```python
from build123d import *

# Parameters (mm, degrees)
SKETCH_3_W           = 10
SKETCH_3_H           = 40
SKETCH_3_W_2         = 25.75
SKETCH_3_H_2         = 10
SKETCH_3_W_3         = 36.25
SKETCH_3_W_4         = 25
EXTRUDE_1_DEPTH      = 1
EXTRUDE_2_DEPTH      = 4
EXTRUDE_2_DEPTH_BACK = 1
SKETCH_5_W           = 25
SKETCH_5_H           = 10
SKETCH_5_W_2         = 10
SKETCH_5_H_2         = 40
EXTRUDE_3_DEPTH      = 2


with BuildPart() as part:
    # 草图3 → 凸台-拉伸1 (new body)
    with BuildSketch(Plane(origin=(0, 0, 0), x_dir=(1, 0, 0), z_dir=(0, 1, 0))):
        with Locations((20, 0)):
            Rectangle(SKETCH_3_W, SKETCH_3_H)
        with Locations((2.125, 0)):
            Rectangle(SKETCH_3_W_2, SKETCH_3_H_2)
        Polygon((-10.75, -5), (-10.75, 5), (-10.75, 25), (-20.75, 25), (-20.75, 5), (-20.75, -5), (-20.75, -25), (-10.75, -25), align=None)
        with Locations((-38.875, 0)):
            Rectangle(SKETCH_3_W_3, SKETCH_3_H_2)
        with Locations((-69.5, 0)):
            Rectangle(SKETCH_3_W_4, SKETCH_3_H_2)
    extrude(amount=EXTRUDE_1_DEPTH)

    # 草图4 → 凸台-拉伸2 (add, two sides)
    with BuildSketch(Plane.XZ) as extrude_2_sk:
        Polygon((14, -21), (26, -21), (26, 21), (14, 21), (14, 6), (-9.75, 6), (-9.75, 26), (-21.75, 26), (-21.75, 6), (-83, 6), (-83, -6), (-21.75, -6), (-21.75, -26), (-9.75, -26), (-9.75, -6), (14, -6), align=None)
        Polygon((15, -20), (25, -20), (25, 20), (15, 20), (15, 5), (-10.75, 5), (-10.75, 25), (-20.75, 25), (-20.75, 5), (-82, 5), (-82, -5), (-20.75, -5), (-20.75, -25), (-10.75, -25), (-10.75, -5), (15, -5), align=None, mode=Mode.SUBTRACT)
    extrude(amount=EXTRUDE_2_DEPTH)
    extrude(extrude_2_sk.sketch, amount=-EXTRUDE_2_DEPTH_BACK)

    # 草图5 → 凸台-拉伸3 (add)
    with BuildSketch(Plane.XZ):
        Polygon((-20.75, 25), (-20.75, 5), (-17, 5), (-17, -5), (-20.75, -5), (-20.75, -25), (-10.75, -25), (-10.75, -5), (-15, -5), (-15, 5), (-10.75, 5), (-10.75, 25), align=None)
        with Locations((-69.5, 0)):
            Rectangle(SKETCH_5_W, SKETCH_5_H)
        with Locations((20, 0)):
            Rectangle(SKETCH_5_W_2, SKETCH_5_H_2)
    extrude(amount=EXTRUDE_3_DEPTH)


solid = part.part
```
The model under review builds one solid part; all positions refer to its coordinate system, in mm. A direction names the side the tool comes from. Coordinates: 2 decimals unless noted, no trailing zeros. Order: outer loops, then holes, each group sorted by start corner. A loop starts at its lowest first (then second) coordinate and runs counter-clockwise, first axis right, second up. Notation, with made-up numbers: (25.5, -11.75) -> (40.5, -11.75) arc R17 cw to (40.5, 15.25) -> close; hole circle Ø3 at (84, 26.5). An arc over 180 degrees is marked (long way). Answer in a Markdown table with one row per item. Add a question column.
Item 1: Machinability: for faces 1 (the flat face through (14, -2, 14)), 2 (the flat face through (14, -2, -13)), 3 (the flat face through (-16, -2, 0)), which of the approach directions +Z, -Z, +X, -X, +Y, -Y give a long, thin tool a straight path to every point of the face, cutting with its end or side? Answer none if there is none.
Item 2: We need section D-D on z = 3. Write out the cut boundary in (x, y), plus the area to 3 significant figures.
Item 3: We need section C-C on x = 16.5. Write out the cut boundary in (y, z), plus the area to 3 significant figures.
Item 4: We need section A-A on z = 15.5. Write out the cut boundary in (x, y), plus the area to 3 significant figures.
Item 5: Clearance check with flat-ended pins moving along their axes: pin 1 (0.6 mm diameter, centred on y = -2.5, z = -6.5, fed in from -X); pin 2 (8 mm diameter, centred on x = 20.5, z = -7, fed in from -Y); pin 3 (2 mm diameter, centred on x = 22.5, y = -3.5, fed in from +Z). State where each tip first meets the part, or that it passes through.
Item 6: To check wall thickness, follow probe 1 along X at (y, z) = (-2.05, -13.5); probe 2 along X at (y, z) = (-3.65, 20.5); probe 3 along Z at (x, y) = (-24, -3.3). State the ranges of each line that lie inside material, in increasing order.
Item 7: Mouldability with a two-part tool opening along Z and no side actions: class faces 4 (the flat face through (15, -3, 13)), 5 (the flat face through (26, -2, 0)), 6 (the flat face through (2, -2, 6)) as +Z half, -Z half, draft (parallel to the pull), parting line (faces both ways), or undercut.
Final values:
| question | item | result |
|---|---|---|
| 1 | face 1 | +Z, +Y, -Y |
| 1 | face 2 | -Z, +Y, -Y |
| 1 | face 3 | -Y |
| 2 | outline | (-83, -4) -> (-82, -4) -> (-82, -2) -> (-57, -2) -> (-57, 0) -> (-17, 0) -> (-17, -2) -> (-15, -2) -> (-15, 0) -> (15, 0) -> (15, -2) -> (25, -2) -> (25, -4) -> (26, -4) -> (26, 1) -> (-83, 1) -> close |
| 2 | area | 191 mm2 |
| 3 | outline | (-4, -21) -> (1, -21) -> (1, 21) -> (-4, 21) -> (-4, 20) -> (-2, 20) -> (-2, -20) -> (-4, -20) -> close |
| 3 | area | 130 mm2 |
| 4 | outline | (-21.75, -4) -> (-20.75, -4) -> (-20.75, -2) -> (-10.75, -2) -> (-10.75, -4) -> (-9.75, -4) -> (-9.75, 1) -> (-21.75, 1) -> close; (14, -4) -> (15, -4) -> (15, -2) -> (25, -2) -> (25, -4) -> (26, -4) -> (26, 1) -> (14, 1) -> close |
| 4 | area | 80.0 mm2 |
| 5 | pin 1 | stops at x = -21.75 |
| 5 | pin 2 | stops at y = -2 |
| 5 | pin 3 | stops at z = 21 |
| 6 | probe 1 | x = -21.75 to -20.75, -10.75 to -9.75, 14 to 15, 25 to 26 |
| 6 | probe 2 | x = -21.75 to -20.75, -10.75 to -9.75, 14 to 26 |
| 6 | probe 3 | z = -6 to -5, 5 to 6 |
| 7 | face 4 | undercut |
| 7 | face 5 | draft |
| 7 | face 6 | +Z half |
